Read the model definition and answer for the solid it produces. Units are mm, in the model's axes. Coordinates: 2 decimals unless noted, no trailing zeros. Loops run counter-clockwise (first coordinate to the right, second up) from the corner with the lowest first, then second, coordinate; pieces in that order, holes last. Notation, with made-up numbers: (87, 9) -> (96, 9) arc R20 cw to (96, 28) -> close; hole circle Ø7 at (76.5, 57.25). An arc over 180 degrees is marked (long way). Answer in a Markdown table with one row per item.
```python
from build123d import *

# Parameters (mm, degrees)
SKETCH002_W = 9
SKETCH002_H = 2.65
SKETCH_R    = 0.55
SKETCH003_W = 2.25
SKETCH003_H = 0.02


with BuildPart() as revolution:
    # Sketch002 → Revolution (revolve)
    with BuildSketch(Plane.XZ):
        with Locations((6.35, 4.475)):
            Rectangle(SKETCH002_W, SKETCH002_H)
    revolve(axis=Axis((1.85, 0, 3.15), (1, 0, 0)))


with BuildPart() as sweep_body:
    # Sweep: sweep along a path in Sketch001
    with BuildLine(Plane.XZ) as sweep_path:
        Line((0, -2.5), (0, 2.05))
        ThreePointArc((0, 2.05), (0.322183, 2.827817), (1.1, 3.15))
        Line((1.1, 3.15), (11.6, 3.15))
        ThreePointArc((11.6, 3.15), (12.377817, 2.827817), (12.7, 2.05))
        Line((12.7, 2.05), (12.7, -2.5))
    # Sketch → Sweep (sweep)
    with BuildSketch(Plane.XY.offset(-2)):
        Circle(SKETCH_R)
    sweep(path=sweep_path.line)


with BuildPart() as obj1:
    # Sketch003 → Revolution001 (revolve)
    with BuildSketch(Plane.XZ):
        with Locations((4.325, 5.8)):
            Rectangle(SKETCH003_W, SKETCH003_H)
    revolve(axis=Axis((0, 0, 3.15), (1, 0, 0)))

    add(revolution.part)
    add(sweep_body.part)


solid = obj1.part
```
1. Given pin 1 Ø2 at (x, z) = (1.5, 3) entering from +Y; pin 2 Ø3 at (x, y) = (11, 1.5) entering from +Z; pin 3 Ø3 at (y, z) = (-1, 0.5) entering from -X; pin 4 Ø1.5 at (x, y) = (6, -1.5) entering from +Z, each flat-ended and moving along its own axis, determine where each tip first touches the part or whether it passes through.
A:
| item | result |
|---|---|
| pin 1 | stops at y = 2.65 |
| pin 2 | stops at z = 5.8 |
| pin 3 | stops at x = -0.55 |
| pin 4 | stops at z = 5.69 |
2. Find the intervals of material crossed by probe 1 along X at (y, z) = (-0.1, -0.5); probe 2 along X at (y, z) = (-1.45, 2.5); probe 3 along Z at (x, y) = (8.75, -0.1), in increasing order.
A:
| item | result |
|---|---|
| probe 1 | x = -0.54 to 0.54, 12.16 to 13.24 |
| probe 2 | x = 1.85 to 10.85 |
| probe 3 | z = 0.5 to 5.8 |
3. A cutting plane is placed at C-C on x = 7. Give the vertices of the cut face in (y, z), and give its area (3 significant figures).
A:
| item | result |
|---|---|
| outline | circle Ø5.3 at (0, 3.15) |
| area | 22.1 mm2 |
4. The mould has two halves that part along X. Classify faces 1 (the cylindrical face through (0.525, 0.165, -0.193)), 2 (the flat face through (0, 0, -2.5)): pulls with the +X half, pulls with the -X half, needs draft (parallel to the pull), parting line crosses it, or undercut.
A:
| item | result |
|---|---|
| face 1 | undercut |
| face 2 | needs draft |
